Could you check a few things on this model? Use its own coordinates, in mm. Face numbers are marked on the shaded views. A direction names the side the tool comes from. Give positions to 0.01 mm unless a question says otherwise; leave off trailing zeros. Loops run counter-clockwise (first coordinate to the right, second up) from the corner with the lowest first, then second, coordinate; pieces in that order, holes last. Notation, with made-up numbers: (40, 83.25) - (64, 83.25) arc R16 ccw to (64, 100.25) - close; hole circle Ø5 at (57.5, 65.5). An arc over 180 degrees is marked (long way). Use CSV: the item, a comma, the result in double quotes.
Autodesk Inventor part; units mm, degrees
ref_plane "YZ Plane" through (0, 0, 0) normal (1, 0, 0) x (0, 1, 0)
ref_plane "XZ Plane" through (0, 0, 0) normal (0, 1, 0) x (-1, 0, 0)
ref_plane "XY Plane" through (0, 0, 0) normal (0, 0, 1) x (1, 0, 0)
sketch "Sketch1" plane through (0, 0, 0) normal (0, 0, 1) x (1, 0, 0)
  circle A0 centre (0, 0) radius 2.5
  dimension "d0" = 5
extrude "Extrusion1" add sketch "Sketch1" along normal blind 5.1
sketch "Sketch2" plane through (0, 0, 0) normal (0, 0, -1) x (-1, 0, 0)
  circle A0 centre (0, 0) radius 2.5
  arc A1 (-0.031716, 2.999832) -> (2.751366, 1.195821) centre (0, 0) ccw
  line L0 (-0.031716, 2.999832) -> (2.751366, 1.195821)
  dimension "d3" = 6
extrude "Extrusion2" add sketch "Sketch2" along normal blind 1 contours A0 | L0 A1
sketch "Sketch4" plane through (0, 0, 0) normal (0, 1, 0) x (-1, 0, 0)
  line L0 (0, 0) -> (0, 10.583317)
  arc A0 (0, 7.5) -> (-2.5, 5) centre (0, 5) ccw
  line L1 (-2.5, 5) -> (0, 5)
  dimension "d11" = 2.5
  dimension "d12" = 5
revolve "Revolution1" add sketch "Sketch4" angle 360 about axis through (0, 0, 0) along (0, 0, 1)
sketch "Sketch5" plane through (0, 0, 0) normal (1, 0, 0) x (0, 1, 0)
  line L0 (-2.165084, -1) -> (-2.915084, -1.75)
  line L1 (-2.915084, -1.75) -> (-2.915084, -3.85)
  line L2 (-2.915084, -3.85) -> (-2.165084, -3.85)
  line L3 (-2.165084, -3.85) -> (-2.165084, -3.75)
  line L4 (-2.165084, -3.75) -> (-0.375084, -3.75)
  line L5 (-0.375084, -3.75) -> (-0.375084, -3.85)
  line L6 (-0.375084, -3.85) -> (0.374916, -3.85)
  line L7 (0.374916, -3.85) -> (0.374916, -3.75)
  line L8 (0.374916, -3.75) -> (2.164916, -3.75)
  line L9 (2.164916, -3.75) -> (2.164916, -3.85)
  line L10 (2.164916, -3.85) -> (2.914916, -3.85)
  line L11 (2.914916, -3.85) -> (2.914916, -1.75)
  line L12 (2.914916, -1.75) -> (2.334916, -1)
  line L13 (2.334916, -1) -> (-2.165084, -1)
  line L14 (2.999832, -1) -> (-3, -1)
  line L15 (-0.000084, -1) -> (-0.000084, -3.532862)
  point P0 (0, 0)
  point P1 (1.195821, -1)
  dimension "d14" = 0.75
  dimension "d15" = 0.75
  dimension "d16" = 0.75
  dimension "d17" = 2.54
  dimension "d18" = 2.54
  dimension "d19" = 2.75
  dimension "d20" = 4.5
  dimension "d21" = 0.75
  dimension "d22" = 0.75
  dimension "d23" = 0.1
  dimension "d24" = 0
  dimension "d25" = 0.375
extrude "Extrusion3" add sketch "Sketch5" along normal mid plane 0.75
sketch "Sketch6" plane through (0.375, -0.375084, -3.85) normal (0, 0, -1) x (-1, 0, 0)
  line L0 (0, 0) -> (0.75, 0.75)
  line L1 (0.75, 0) -> (0, 0.75)
  circle A0 centre (0.375, 0.375084) radius 0.375
  point P0 (0.375, 0.375084)
sketch "Sketch7" plane through (0.375, 2.164916, -3.85) normal (0, 0, -1) x (-1, 0, 0)
  line L0 (0, 0.75) -> (0.75, 0)
  line L1 (0.75, 0.75) -> (0, 0)
  circle A0 centre (0.375, 0.375) radius 0.375
  point P0 (0.375, -2.164916)
sketch "Sketch8" plane through (0.375, -2.915084, -3.85) normal (0, 0, -1) x (-1, 0, 0)
  line L0 (0, 0.75) -> (0.75, 0)
  line L1 (0.75, 0.75) -> (0, 0)
  circle A0 centre (0.375, 0.375) radius 0.375
  point P0 (0.375, 2.915084)
extrude "Extrusion4" add sketch "Sketch8" along normal blind 5
extrude "Extrusion5" add sketch "Sketch6" along normal blind 5
extrude "Extrusion6" add sketch "Sketch7" along normal blind 5
properties part number "LED"
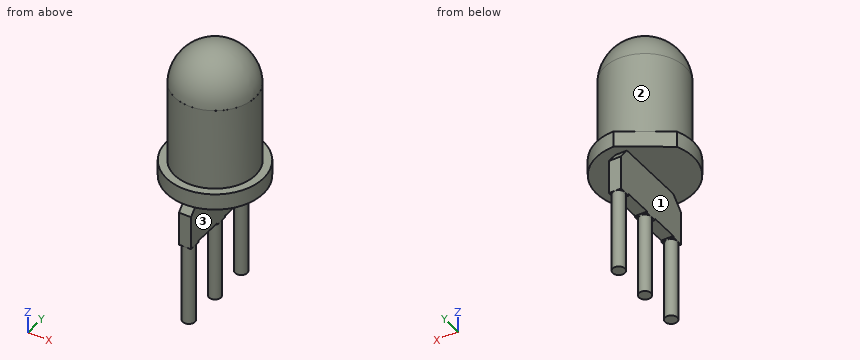
1) I'm going to push flat-ended pins straight in: P1, Ø1.8, axis at x = 1, y = 1, coming from the +Z side; P2, Ø3, axis at x = -2, y = 1.5, coming from the -Z side; P3, Ø0.6, axis at x = 0, y = -1, coming from the -Z side. Where does each tip first touch, or does it pass through?
Answer below:
P1,"stops at z = 7.45"
P2,"stops at z = -1"
P3,"stops at z = -3.75"
2) I need wall thicknesses on line 1 along Y through (x, z) = (-0.1, 3.5); line 2 along Z through (x, y) = (-2.65, -0.8); line 3 along Z through (x, y) = (1.95, 0.1). Which ranges of each line are inside material? Lowest first, please.
Answer below:
line 1,"y = -2.5 to 2.5"
line 2,"z = -1 to 0"
line 3,"z = -1 to 6.56"
3) Suppose I cut it at A-A (z = -4). Please give me the cut outline in (x, y) (3 decimals), plus the area to 3 significant figures.
Answer below:
outline,"circle Ø0.75 at (0, -2.54); circle Ø0.75 at (0, 0); circle Ø0.75 at (0, 2.54)"
area,"1.33 mm2"
4) Which directions (+Z, -Z, +X, -X, +Y, -Y) give clear straight access to the entire face, cutting with the end or side of a thin tool? Please do the marked faces 1, 2 and 3.
Answer below:
face 1,"-Z, -X, +Y, -Y"
face 2,"+Z"
face 3,"-Z, +X, +Y, -Y"
